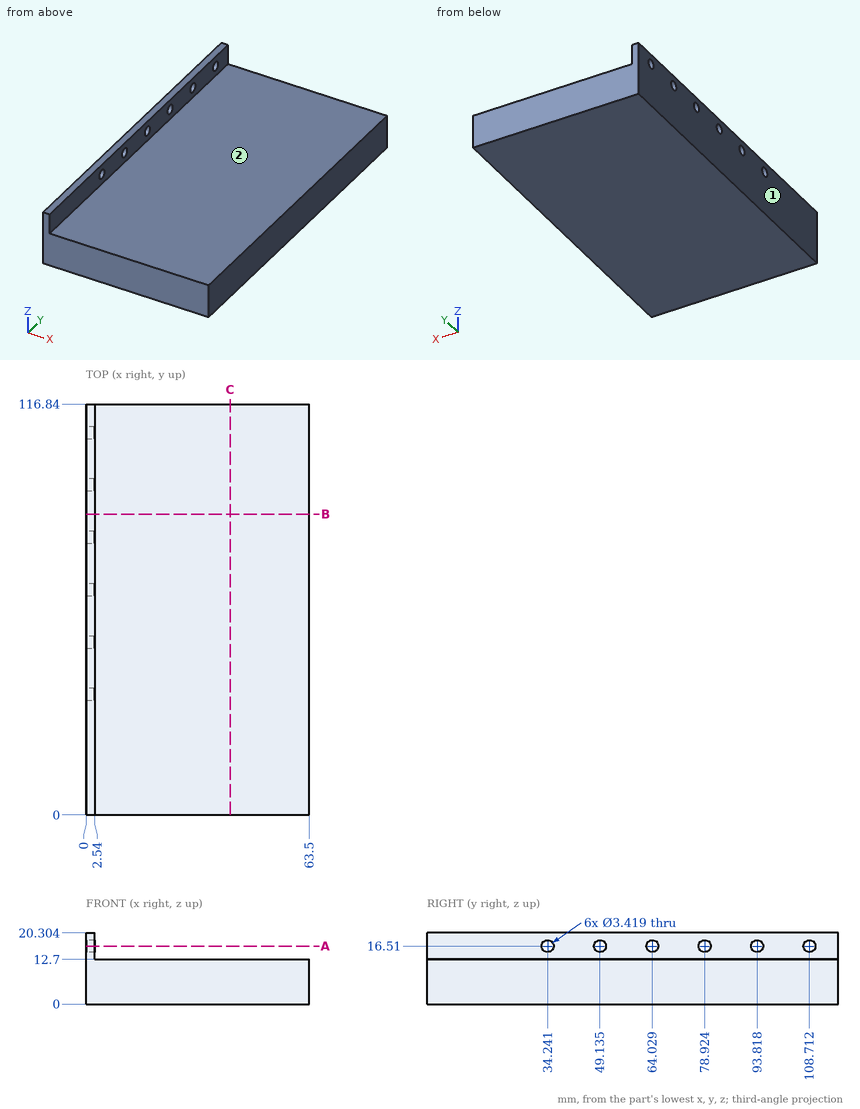
Study the drawing (mm; zero at the part's minimum x, y, z) and answer. A direction names the side the tool comes from. Coordinates: 2 decimals unless noted, no trailing zeros. Write each loop counter-clockwise with the first axis right and the second up, starting at its lowest first coordinate (ties: lowest second). Pieces come first, ordered by that corner, then holes.
Q1. A cutting plane is placed at A-A, the plane z = 16.51. State how many separate pieces and enclosed holes the cut face has.
Q2. Each of these flat-tipped pins is pushed along its axis until it touches: pin 1 Ø3 at (y, z) = (49.14, 16.51) entering from -X; pin 2 Ø18.5 at (x, y) = (36.5, 64) entering from +Z. Where does it stop, or does it pass through?
Q3. Find the intervals of material crossed by line 1 (Z direction, x = 48.5, y = 67.5); line 2 (X direction, y = 8.5, z = 16.5), in increasing order.
Q4. A cutting plane is placed at B-B, the plane y = 85.5. Give the vertices of the cut face in (x, z), then the cut area to 3 significant figures.
Q5. A cutting plane is placed at C-C, the plane x = 41. Give the vertices of the cut face in (y, z), then the cut area to 3 significant figures.
Q6. Which of the six approach directions +Z, -Z, +X, -X, +Y, -Y give full straight-line access (tool end or side, diameter ignored) to the marked faces 1 and 2?
Findings below:
1. separate pieces: 7
1. enclosed holes: 0
2. pin 1: passes through
2. pin 2: stops at z = 12.7
3. line 1: z = 0 to 12.7
3. line 2: x = 0 to 2.54
4. outline: (0, 0) - (63.5, 0) - (63.5, 12.7) - (2.54, 12.7) - (2.54, 20.3) - (0, 20.3) - close
4. area: 826 mm2
5. outline: (0, 0) - (116.84, 0) - (116.84, 12.7) - (0, 12.7) - close
5. area: 1,480 mm2
6. face 1: +Z, -Z, -X, +Y, -Y
6. face 2: +Z, +X, +Y, -Y
